```python
from build123d import *

# Parameters (mm, degrees)
SKETCH1_W               = 90
SKETCH1_H               = 90
BOSS_EXTRUDE1_DEPTH     = 20
CUT_EXTRUDE1_DEPTH      = 67.708320321
CUT_EXTRUDE1_DEPTH_BACK = 67.708320321
CUT_EXTRUDE2_DEPTH      = 67.708320486
CUT_EXTRUDE2_DEPTH_BACK = 67.708320486
CUT_EXTRUDE13_DEPTH     = 10
BOSS_EXTRUDE5_START     = 6.5
BOSS_EXTRUDE5_DEPTH     = 26.5
BOSS_EXTRUDE7_START     = -25
SKETCH26_W              = 3
SKETCH26_H              = 18.966666926
BOSS_EXTRUDE7_DEPTH     = 20
CUT_EXTRUDE23_START     = 25
SKETCH28_R              = 1.55
CUT_EXTRUDE23_DEPTH     = 10
CUT_EXTRUDE24_START     = 35
CUT_EXTRUDE24_DEPTH     = 10


with BuildPart() as part:
    # Sketch1 → Boss-Extrude1 (new body)
    with BuildSketch(Plane.XY):
        Rectangle(SKETCH1_W, SKETCH1_H)
    extrude(amount=BOSS_EXTRUDE1_DEPTH)

    # Sketch2 → Cut-Extrude1 (cut, two sides)
    with BuildSketch(Plane(origin=(0, 0, 0), x_dir=(0, 0, -1), z_dir=(1, 0, 0))) as cut_extrude1_sk:
        with BuildLine():
            Line((0, -45), (0, 45))
            Line((0, 45), (-17.5, 45))
            add(Edge.make_bspline(
                [(-17.5, 45), (1.11526928, 18.330109849), (-2.773030501, -17.812088562), (-17.5, -45)],
                knots=[0, 0, 0, 0, 1, 1, 1, 1], degree=3))
            Line((-17.5, -45), (0, -45))
        make_face()
        with BuildLine():
            add(Edge.make_bspline(
                [(-20, 45), (3.100953483, 4.754137608), (-20, -45)],
                knots=[0, 0, 0, 1, 1, 1], degree=2))
            Line((-20, -45), (-20, 45))
        make_face()
    extrude(amount=CUT_EXTRUDE1_DEPTH, mode=Mode.SUBTRACT)
    extrude(cut_extrude1_sk.sketch, amount=-CUT_EXTRUDE1_DEPTH_BACK, mode=Mode.SUBTRACT)

    # Sketch3 → Cut-Extrude2 (cut, two sides)
    with BuildSketch(Plane.XY) as cut_extrude2_sk:
        with BuildLine():
            ThreePointArc((5.952933229, -30.681551854), (0, -33.619470534), (-5.952933229, -30.681551854))
            Line((-5.952933229, -30.681551854), (-14.882333073, -19.02982596))
            add(Edge.make_bspline(
                [(-14.882333073, -19.02982596), (-33.37703632, -2.819308001), (-57.954503959, 42.329469412), (-9.638427065, 45)],
                knots=[0, 0, 0, 0, 0.942687649, 0.942687649, 0.942687649, 0.942687649], degree=3))
            Line((-9.638427065, 45), (-45, 45))
            Line((-45, 45), (-45, -45))
            Line((-45, -45), (45, -45))
            Line((45, -45), (45, 45))
            Line((45, 45), (9.638427065, 45))
            add(Edge.make_bspline(
                [(14.882333073, -19.02982596), (33.37703632, -2.819308001), (57.954503959, 42.329469412), (9.638427065, 45)],
                knots=[0, 0, 0, 0, 0.942687649, 0.942687649, 0.942687649, 0.942687649], degree=3))
            Line((14.882333073, -19.02982596), (5.952933229, -30.681551854))
        make_face()
    extrude(amount=CUT_EXTRUDE2_DEPTH, mode=Mode.SUBTRACT)
    extrude(cut_extrude2_sk.sketch, amount=-CUT_EXTRUDE2_DEPTH_BACK, mode=Mode.SUBTRACT)

    # Sketch15 → Cut-Extrude13 (cut)
    with BuildSketch(Plane(origin=(0, 0, 0), x_dir=(0, 0, -1), z_dir=(1, 0, 0))):
        Polygon((-6.544274822, -14.084003466), (-5.916371018, -10.261977823), (-5.185386391, -14.084003466), align=None)
    extrude(amount=CUT_EXTRUDE13_DEPTH, mode=Mode.SUBTRACT)

    # Sketch24 → Boss-Extrude5 (add)
    with BuildSketch(Plane.XY.offset(BOSS_EXTRUDE5_START)):
        Polygon((-15.802792048, 6.336123183), (-6.155905041, -11.183510692), (-3.52795996, -9.736477641), (-13.174846966, 7.783156234), align=None)
    extrude(amount=BOSS_EXTRUDE5_DEPTH)

    # Sketch26 → Boss-Extrude7 (add)
    with BuildSketch(Plane(origin=(0, 0, 0), x_dir=(0, 0, -1), z_dir=(1, 0, 0)).offset(BOSS_EXTRUDE7_START)):
        with Locations((-31.5, -1.700177229)):
            Rectangle(SKETCH26_W, SKETCH26_H)
    extrude(amount=BOSS_EXTRUDE7_DEPTH)

    # Sketch28 → Cut-Extrude23 (cut)
    with BuildSketch(Plane.XY.offset(CUT_EXTRUDE23_START)):
        with Locations((-20.256840538, 4.115140616)):
            Circle(SKETCH28_R)
        with BuildLine():
            Line((-18.706840538, -7.619333671), (-18.706840538, 4.115140616))
            ThreePointArc((-18.706840538, 4.115140616), (-20.256840538, 2.565140616), (-21.806840538, 4.115140616))
            Line((-21.806840538, 4.115140616), (-21.806840538, -7.619333671))
            ThreePointArc((-21.806840538, -7.619333671), (-20.256840538, -6.069333671), (-18.706840538, -7.619333671))
        make_face()
        with Locations((-20.256840538, -7.619333671)):
            Circle(SKETCH28_R)
    extrude(amount=CUT_EXTRUDE23_DEPTH, mode=Mode.SUBTRACT)

    # Sketch29 → Cut-Extrude24 (cut)
    with BuildSketch(Plane.XY.offset(CUT_EXTRUDE24_START)):
        Polygon((-3.77618872, 7.783156234), (-3.52795996, -9.736477641), (-13.688384135, 7.783156234), align=None)
        Polygon((-7.35673341, -11.956955683), (-3.65207434, -11.956955683), (-3.52795996, -9.736477641), align=None)
    extrude(amount=-CUT_EXTRUDE24_DEPTH, mode=Mode.SUBTRACT)


solid = part.part
```
Model file for the job. Use its own axes, mm. A direction names the side the tool comes from. Coordinates: 2 decimals unless noted, no trailing zeros. Order: outer loops, then holes, each group sorted by start corner. A loop starts at its lowest first (then second) coordinate and runs counter-clockwise, first axis right, second up. Notation, with made-up numbers: (43.25, -19.5) -> (53.25, -19.5) arc R24 ccw to (53.25, 16.5) -> close; hole circle Ø5 at (40.25, -35). An arc over 180 degrees is marked (long way). Answer as a JSON object with one key per item and string values. Group by question number.
1) Drill centre lines: L1, parallel to Y at x = -14, z = 17.75; L2, parallel to Z at x = -21, y = 1.5; L3, parallel to Z at x = -8.5, y = 22.5. Where is each one in solid material? Low to high.
2) Pull direction X, two halves, no side cores. Call faces 5 (the face through (-14, -4, 33)), 6 (the face through (-25, -2, 32)), 7 (the face through (-18.707, -2, 31)): +X half, -X half, draft (parallel to the pull), parting line (faces both ways), or undercut.
3) Which spindle directions (+Z, -Z, +X, -X, +Y, -Y) get a long thin tool onto all of the face, cutting with end or side? Do faces 1 (the face through (-16, -11.184, 32)), 2 (the face through (-11.047, -2.301, 19.045)), 3 (the face through (-19, 7.783, 32)), 4 (the face through (-20.223, 5.665, 31.479)). Say none if no direction does.
4) Cut at A-A, the plane z = 21.5. Write the cut outline in (x, y), then the cut area to 3 significant figures.
5) Flat gauge pins, fed straight in: pin 1 (8 mm diameter, centred on y = 15.5, z = 25, fed in from +X); pin 2 (4 mm diameter, centred on x = 13.5, y = -14.5, fed in from +Z); pin 3 (12 mm diameter, centred on y = 33, z = 14.5, fed in from -X); pin 4 (2.5 mm diameter, centred on x = -20, z = 31, fed in from +Y). Where does each tip first touch, or does it go through?
6) Cut at B-B, the plane z = 27.75. Write the cut outline in (x, y), then the cut area to 3 significant figures.
Check values:
{
 "1": {"L1": "y = 3.06 to 7.33, 40.84 to 44.62", "L2": "z = 4.97 to 8.45", "L3": "z = 7.31 to 10.88"},
 "2": {"face 5": "draft", "face 6": "-X half", "face 7": "undercut"},
 "3": {"face 1": "+Z, +X, -X, -Y", "face 2": "-X", "face 3": "+Z, +X, -X, +Y", "face 4": "+Z"},
 "4": {"outline": "(-15.8, 6.34) -> (-6.16, -11.18) -> (-3.53, -9.74) -> (-13.17, 7.78) -> close", "area": "60.0 mm²"},
 "5": {"pin 1": "passes through", "pin 2": "stops at z = 10.4", "pin 3": "stops at x = -37.48", "pin 4": "stops at y = 7.78"},
 "6": {"outline": "(-15.8, 6.34) -> (-6.16, -11.18) -> (-3.53, -9.74) -> (-13.56, 7.57) -> close", "area": "55.6 mm²"}
}
